from build123d import *

# Parameters (mm, degrees)
F0_W     = 37
F0_H     = 4
F1_DEPTH = 20
F3_DEPTH = 8
F5_DEPTH = 37
F7_D     = 4.4
F7_DEPTH = 10
F7_TIP   = 1.3218933619


with BuildPart() as f1:
    # F0 (on Front) → F1 (new body)
    with BuildSketch(Plane.XZ):
        with Locations((0, 2)):
            Rectangle(F0_W, F0_H)
    extrude(amount=F1_DEPTH)

    # F2 (on face) → F3 (join)
    with BuildSketch(Plane.XZ.offset(20)):
        Polygon((0.754779164, 4.7), (0.5, 4), (2, 4), (1.745220836, 4.7), align=None)
        Polygon((-2, 4), (-0.5, 4), (-0.754779164, 4.7), (-1.745220836, 4.7), align=None)
        Polygon((4.5, 4), (4.245220836, 4.7), (3.254779164, 4.7), (3, 4), align=None)
        Polygon((7, 4), (6.745220836, 4.7), (5.754779164, 4.7), (5.5, 4), align=None)
        Polygon((9.5, 4), (9.245220836, 4.7), (8.254779164, 4.7), (8, 4), align=None)
        Polygon((12, 4), (11.745220836, 4.7), (10.754779164, 4.7), (10.5, 4), align=None)
        Polygon((14.5, 4), (14.245220836, 4.7), (13.254779164, 4.7), (13, 4), align=None)
        Polygon((17, 4), (16.745220836, 4.7), (15.754779164, 4.7), (15.5, 4), align=None)
        Polygon((-9.5, 4), (-8, 4), (-8.254779164, 4.7), (-9.245220836, 4.7), align=None)
        Polygon((-17, 4), (-15.5, 4), (-15.754779164, 4.7), (-16.745220836, 4.7), align=None)
        Polygon((-5.754779164, 4.7), (-6.745220836, 4.7), (-7, 4), (-5.5, 4), align=None)
        Polygon((-4.5, 4), (-3, 4), (-3.254779164, 4.7), (-4.245220836, 4.7), align=None)
        Polygon((-14.5, 4), (-13, 4), (-13.254779164, 4.7), (-14.245220836, 4.7), align=None)
        Polygon((-10.754779164, 4.7), (-11.745220836, 4.7), (-12, 4), (-10.5, 4), align=None)
    extrude(amount=-F3_DEPTH)

    # F4 (on face) → F5 (join, through all)
    with BuildSketch(Plane.YZ.offset(18.5)):
        with BuildLine():
            Line((-2.6, 4), (0, 4))
            ThreePointArc((0, 4), (-1.3, 5.3), (-2.6, 4))
        make_face()
    extrude(amount=-F5_DEPTH)

    # F7
    with Locations(Plane(origin=(0, 0, 0), x_dir=(1, 0, 0), z_dir=(0, 0, -1))):
        with Locations((10, 9), (-10, 9)):
            Hole(F7_D / 2, depth=F7_DEPTH)
            with Locations((0, 0, -(F7_DEPTH + F7_TIP / 2))):  # 118° drill point
                Cone(0, F7_D / 2, F7_TIP, mode=Mode.SUBTRACT)


solid = f1.part
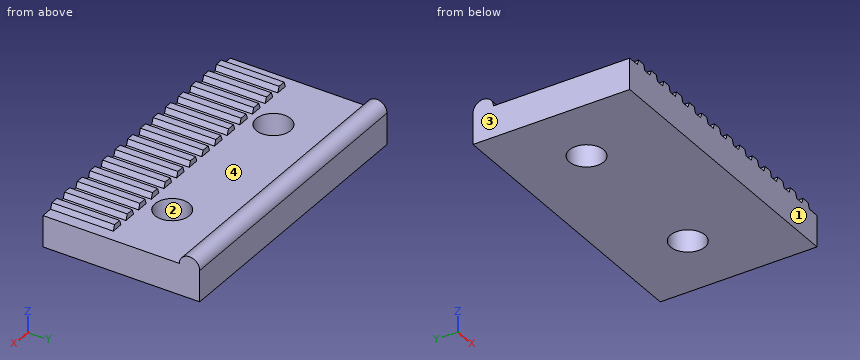
Design review of the part built by this model. Coordinates are the model's own, in mm. Face numbers are marked on the shaded views. Coordinates: 2 decimals unless noted, no trailing zeros. Order: outer loops, then holes, each group sorted by start corner. A loop starts at its lowest first (then second) coordinate and runs counter-clockwise, first axis right, second up. Notation, with made-up numbers: M -30.75,71.5 L 4.25,71.5 A23 cw 4.25,106.5 Z; hole C 37.5,0 d7. An arc over 180 degrees is marked long. Use a Markdown table: item, result.
(1) Add section A-A (x = -10). Give the boundary of the cut face in (y, z).
Worked answers:
| item | result |
|---|---|
| outline | M -20,0 L -11.2,0 L -11.2,4 L -20,4 Z; M -6.8,0 L 0,0 L 0,4 A1.3 ccw -2.6,4 L -6.8,4 Z |
(2) Wall thickness on probe 1 along Y at (x, z) = (1.5, 4.15); probe 2 along X at (y, z) = (-9, 2.15); probe 3 along X at (y, z) = (-8.5, 1.65): over which ranges is each line inside the solid? List them lowest first.
Worked answers:
| item | result |
|---|---|
| probe 1 | y = -20 to -12, -2.59 to -0.01 |
| probe 2 | x = -18.5 to -12.2, -7.8 to 7.8, 12.2 to 18.5 |
| probe 3 | x = -18.5 to -12.14, -7.86 to 7.86, 12.14 to 18.5 |
(3) Add section B-B (y = -10.5). Give the boundary of the cut face in (x, z), then the cut area to 3 significant figures.
Worked answers:
| item | result |
|---|---|
| outline | M -18.5,0 L -11.61,0 L -11.61,4 L -18.5,4 Z; M -8.39,0 L 8.39,0 L 8.39,4 L -8.39,4 Z; M 11.61,0 L 18.5,0 L 18.5,4 L 11.61,4 Z |
| area | 122 mm2 |
(4) Draft analysis for pull direction X (two halves, no side actions). For the marked faces 1, 2, 3 and 4, state which applies: released by +X, released by -X, zero draft, split by the parting line, or undercut.
Worked answers:
| item | result |
|---|---|
| face 1 | zero draft |
| face 2 | undercut |
| face 3 | released by -X |
| face 4 | undercut |
(5) Add section C-C (z = 0.5). Give the boundary of the cut face in (x, y), then the cut area to 3 significant figures.
Worked answers:
| item | result |
|---|---|
| outline | M -18.5,-20 L 18.5,-20 L 18.5,0 L -18.5,0 Z; hole C -10,-9 d4.4; hole C 10,-9 d4.4 |
| area | 710 mm2 |
(6) For P1, Ø0.8, axis at x = -3.5, z = 4.5, coming from the +Y side; P2, Ø0.5, axis at x = 16, y = -18, coming from the +Z side, all flat-tipped, find the tip position at first contact; note any pin that passes through.
Worked answers:
| item | result |
|---|---|
| P1 | stops at y = 0 |
| P2 | stops at z = 4.7 |
